Design review of the part built by this model. Coordinates are the model's own, in mm. A direction names the side the tool comes from. Give positions to 0.01 mm unless a question says otherwise; leave off trailing zeros. Loops run counter-clockwise (first coordinate to the right, second up) from the corner with the lowest first, then second, coordinate; pieces in that order, holes last.
from build123d import *

# Parameters (mm, degrees)
F0_R     = 7
F1_DEPTH = 12
F0_R_2   = 18.6535272591
F2_DEPTH = 12
F3_R     = 5
F5_W     = 10.5
F5_H     = 30
F6_DEPTH = 15
F7_R     = 3


# Not quite as in the source:
# - a feature names something its author has since deleted; it is built from what else it names


with BuildPart() as f1:
    # F0 (on Top) → F1 (new body)
    with BuildSketch(Plane.XY):
        Circle(F0_R)
        Polygon((1.8, 1), (4.5, 1), (4.5, -1), (1.8, -1), (-1.8, -1), (-4.5, -1), (-4.5, 1), (-1.8, 1), (-1.8, 4.32), (1.8, 4.32), align=None, mode=Mode.SUBTRACT)
    extrude(amount=F1_DEPTH)

    # F0 (on Top) → F2 (join)
    with BuildSketch(Plane.XY):
        Circle(F0_R_2)
        Circle(F0_R, mode=Mode.SUBTRACT)
    extrude(amount=F2_DEPTH)

    # F3
    f3_edges = [f1.edges().sort_by_distance(p)[0] for p in [
        (-18.653527, 0, 12),
    ]]
    fillet(f3_edges, radius=F3_R)

    # F5 (on offset) → F6 (join)
    with BuildSketch(Plane.XY.offset(7)):
        Rectangle(F5_W, F5_H)
    extrude(amount=F6_DEPTH)

    # F7
    f7_edges = [f1.edges().sort_by_distance(p)[0] for p in [
        (0, 15, 22),
        (-5.25, 0, 22),
        (5.25, 0, 22),
    ]]
    fillet(f7_edges, radius=F7_R)


solid = f1.part
Q1. Take a section at A-A (z = 5). Give the boundary of the cut face in (x, y), plus the area to 3 significant figures.
Results:
outline: circle Ø37.31 at (0, 0); hole (-4.5, -1) - (4.5, -1) - (4.5, 1) - (1.8, 1) - (1.8, 4.32) - (-1.8, 4.32) - (-1.8, 1) - (-4.5, 1) - close
area: 1,060 mm2
Q2. Take a section at B-B (y = 0). Give the boundary of the cut face in (x, z).
Results:
outline: (-18.65, 0) - (-4.5, 0) - (-4.5, 7) - (4.5, 7) - (4.5, 0) - (18.65, 0) - (18.65, 7) arc R5 ccw to (13.65, 12) - (5.25, 12) - (5.25, 19) arc R3 ccw to (2.25, 22) - (-2.25, 22) arc R3 ccw to (-5.25, 19) - (-5.25, 12) - (-13.65, 12) arc R5 ccw to (-18.65, 7) - close
Q3. Draft analysis for pull direction X (two halves, no side actions). For faces 4 (the face through (0, 4.32, 3)), 5 (the face through (0.07, 14.48, 20.69)), 6 (the face through (-5.25, 0, 15)), state which applies: pulls with the +X half, pulls with the -X half, needs draft (parallel to the pull), parting line crosses it, or undercut.
Results:
face 4: undercut
face 5: needs draft
face 6: pulls with the -X half
Q4. Take a section at D-D (z = 18.5). Give the boundary of the cut face in (x, y).
Results:
outline: (-5.25, -15) - (5.25, -15) - (5.25, 15) - (-5.25, 15) - close
Q5. Take a section at C-C (x = 0). Give the boundary of the cut face in (y, z).
Results:
outline: (-18.65, 0) - (-1, 0) - (-1, 7) - (4.32, 7) - (4.32, 0) - (18.65, 0) - (18.65, 7) arc R5 ccw to (15, 11.82) - (15, 19) arc R3 ccw to (12, 22) - (-15, 22) - (-15, 11.82) arc R5 ccw to (-18.65, 7) - close
Q6. Insertion check: pin 1 (3 mm diameter, centred on x = 8, z = 17, fed in from -Y); pin 2 (0.8 mm diameter, centred on x = -3, z = 2.5, fed in from -Y); pin 3 (1.1 mm diameter, centred on x = 0, z = 3.5, fed in from -Y); pin 4 (8.5 mm diameter, centred on x = 2.5, z = 14.5, fed in from +Y). Each pin has a flat end and moves straight along its axis. Give the tip position at first contact, or say it passes through.
Results:
pin 1: passes through
pin 2: stops at y = -18.47
pin 3: stops at y = -18.65
pin 4: stops at y = 17.31
Q7. Wall thickness on line 1 (Y direction, x = -5, z = 13.25); line 2 (Z direction, x = -6, y = 9); line 3 (X direction, y = -9.5, z = 18.5): over which ranges is each line inside the solid? List them lowest first.
Results:
line 1: y = -15 to 15
line 2: z = 0 to 12
line 3: x = -5.25 to 5.25
Q8. Tool access review of faces 1 (the face through (-4.5, 0, 3)), 2 (the face through (8, 0, 12)), 3 (the face through (-9, 0, 12)): name each direction out of +Z, -Z, +X, -X, +Y, -Y from which nothing blocks a thin tool from reaching the whole face with its end or side.
Results:
face 1: -Z
face 2: +Z, +X, +Y, -Y
face 3: +Z, -X, +Y, -Y
